Geometry check sheet. Reference: the model listing, model coordinates, mm. Round coordinates to 2 decimals unless told otherwise and drop trailing zeros. Loops run counter-clockwise (first coordinate to the right, second up) from the corner with the lowest first, then second, coordinate; pieces in that order, holes last. Notation, with made-up numbers: M -10,-6.75 L 24,-6.75 A22 ccw 24,2.25 Z; hole C 38,-6.75 d10. An arc over 180 degrees is marked long. Write item = value, one per line.
Autodesk Inventor part; units mm, degrees
ref_plane "YZ Plane" through (0, 0, 0) normal (1, 0, 0) x (0, 1, 0)
ref_plane "XZ Plane" through (0, 0, 0) normal (0, 1, 0) x (-1, 0, 0)
ref_plane "XY Plane" through (0, 0, 0) normal (0, 0, 1) x (1, 0, 0)
sketch "Sketch1" plane through (0, 0, 0) normal (0, 0, 1) x (1, 0, 0)
  circle A0 centre (0, 0) radius 25
  dimension "d0" = 50
extrude "Extrusion1" add sketch "Sketch1" along normal mid plane 340
sketch "Sketch2" plane through (0, 0, -170) normal (0, 0, -1) x (-1, 0, 0)
  circle A0 centre (0, 0) radius 25
  circle A1 centre (0, 0) radius 9.5
  dimension "d3" = 19
extrude "Extrusion2" cut sketch "Sketch2" against normal blind 555 contours A1
fillet "Fillet1" radius 2 2 edges at (-25, 0, -170) (-25, 0, 170)
properties part number "ADSK-MH-10049" material "Rubber"
(1) Material ranges on line 1 along Y through (x, z) = (-1, 85.5); line 2 along Y through (x, z) = (0, 50.5); line 3 along X through (y, z) = (-3.5, 88.5), recorded low to high. Write a range as from..to.
Result set:
line_1 = -24.98..-9.45, 9.45..24.98
line_2 = -25..-9.5, 9.5..25
line_3 = -24.75..-8.83, 8.83..24.75
(2) Release check for a two-part mould opening along X. For faces 1 (the flat face through (10, 0, -170)), 2 (the cylindrical face through (23.846, 7.509, 2.352)), 3 (the cylindrical face through (-4.38, -8.43, -2.38)) record: released by +X, released by -X, zero draft, split by the parting line, or undercut.
Result set:
face_1 = zero draft
face_2 = split by the parting line
face_3 = undercut
(3) Depth check by flat-ended pin: pin 1 Ø6 at (y, z) = (17.5, 63.5) entering from -X; pin 2 Ø10 at (y, z) = (-14.5, -64.5) entering from +X; pin 3 Ø6 at (y, z) = (-8.5, 133) entering from +X. Enter the tip coordinate at first touch or a pass-through.
Result set:
pin_1 = -20.37
pin_2 = 23.12
pin_3 = 24.39
(4) Sectioned sample at C-C on z = -19.5. Record the cut outline in (x, y).
Result set:
outline = C 0,0 d50; hole C 0,0 d19
(5) Sectioned sample at A-A on y = 0. Record the cut outline in (x, z).
Result set:
outline = M -25,-168 A2 ccw -23,-170 L -9.5,-170 L -9.5,170 L -23,170 A2 ccw -25,168 Z; M 9.5,-170 L 23,-170 A2 ccw 25,-168 L 25,168 A2 ccw 23,170 L 9.5,170 Z
